from build123d import *

# Parameters (mm, degrees)
BOSS_EXTRU_1_DEPTH = 1.9


with BuildPart() as part:
    # Esquisse1 → Boss.-Extru.1 (new body)
    with BuildSketch(Plane.XY):
        with BuildLine():
            Line((103.141629659, -93.104422445), (-104.537862265, -93.104422445))
            add(Edge.make_bspline(
                [(-104.537862265, -93.104422445), (-104.576313156, -93.104422445), (-104.614764048, -93.104422445), (-104.653209533, -93.104125461), (-104.768513557, -93.101452602), (-104.883671631, -93.090761166), (-104.960260867, -93.08067219), (-105.150982063, -93.049552521), (-105.339086356, -93.007455152), (-105.450747192, -92.977883193), (-105.671146078, -92.909389067), (-105.884660771, -92.820748262), (-105.989422935, -92.771633631), (-106.194408631, -92.664300797), (-106.389220526, -92.539730583), (-106.48384332, -92.473274378), (-106.667043194, -92.332296267), (-106.837192824, -92.17573974), (-106.91879647, -92.093784348), (-107.074644208, -91.922954256), (-107.214938405, -91.739155447), (-107.281028071, -91.644254137), (-107.404754439, -91.448928258), (-107.51089869, -91.243516958), (-107.55945325, -91.138557181), (-107.64728317, -90.924663828), (-107.716066547, -90.703891793), (-107.745614057, -90.592075935), (-107.794855636, -90.366164197), (-107.824060167, -90.136851737), (-107.833655342, -90.021622167), (-107.842835855, -89.790570025), (-107.832005382, -89.559439241), (-107.821514669, -89.444212724), (-107.790403383, -89.216374252), (-107.738630165, -88.992714706), (-107.708207682, -88.882559264), (-107.650563592, -88.701220982), (-107.582401802, -88.523090493), (-107.553106564, -88.452964824), (-107.50557398, -88.350258026), (-107.451336724, -88.251263547), (-107.432968479, -88.218893501), (-107.414357288, -88.186657973), (-107.395746098, -88.154422445)],
                knots=[0, 0, 0, 0, 0, 0, 0.027851934, 0.027851934, 0.027851934, 0.083555801, 0.083555801, 0.083555801, 0.167111603, 0.167111603, 0.167111603, 0.250667404, 0.250667404, 0.250667404, 0.334223205, 0.334223205, 0.334223205, 0.417779006, 0.417779006, 0.417779006, 0.501334808, 0.501334808, 0.501334808, 0.584890609, 0.584890609, 0.584890609, 0.66844641, 0.66844641, 0.66844641, 0.752002212, 0.752002212, 0.752002212, 0.835558013, 0.835558013, 0.835558013, 0.918223942, 0.918223942, 0.918223942, 0.973037938, 0.973037938, 0.973037938, 1, 1, 1, 1, 1, 1], degree=5))
            Line((-107.395746098, -88.154422445), (-3.556000135, 91.701293407))
            add(Edge.make_bspline(
                [(-3.556000135, 91.701293407), (-3.53677469, 91.734592855), (-3.517549244, 91.767892304), (-3.498069305, 91.801038579), (-3.43810253, 91.899558363), (-3.371264438, 91.993942462), (-3.324232511, 92.055226199), (-3.201921489, 92.204835765), (-3.071411952, 92.346690177), (-2.989971465, 92.428605318), (-2.820454369, 92.585229289), (-2.636931834, 92.725818035), (-2.542016234, 92.791987415), (-2.346570425, 92.915843818), (-2.141283507, 93.022270761), (-2.036419348, 93.070988402), (-1.822728786, 93.159155091), (-1.602072042, 93.22823073), (-1.490294768, 93.257923864), (-1.264427699, 93.307476918), (-1.035106162, 93.337075852), (-0.919874384, 93.346860527), (-0.688854027, 93.356347766), (-0.457890497, 93.345565733), (-0.342715384, 93.335135327), (-0.113563347, 93.304251593), (0.112022532, 93.253433727), (0.223631661, 93.223114692), (0.443897755, 93.152803282), (0.657090436, 93.063438917), (0.761679759, 93.014133797), (0.96636704, 92.906558284), (1.161116934, 92.781613428), (1.255660668, 92.714914945), (1.437418929, 92.574052545), (1.605227169, 92.41738585), (1.685413339, 92.335961486), (1.813634853, 92.195371099), (1.933819487, 92.047276013), (1.979902479, 91.986842758), (2.045082883, 91.894324933), (2.103695988, 91.797856852), (2.122545148, 91.765764463), (2.141156339, 91.733528935), (2.159767529, 91.701293407)],
                knots=[0, 0, 0, 0, 0, 0, 0.027851934, 0.027851934, 0.027851934, 0.083555801, 0.083555801, 0.083555801, 0.167111603, 0.167111603, 0.167111603, 0.250667404, 0.250667404, 0.250667404, 0.334223205, 0.334223205, 0.334223205, 0.417779006, 0.417779006, 0.417779006, 0.501334808, 0.501334808, 0.501334808, 0.584890609, 0.584890609, 0.584890609, 0.66844641, 0.66844641, 0.66844641, 0.752002212, 0.752002212, 0.752002212, 0.835558013, 0.835558013, 0.835558013, 0.918223942, 0.918223942, 0.918223942, 0.973037938, 0.973037938, 0.973037938, 1, 1, 1, 1, 1, 1], degree=5))
            Line((2.159767529, 91.701293407), (105.997013492, -88.150092318))
            add(Edge.make_bspline(
                [(105.997013492, -88.150092318), (105.997513492, -88.150958343), (105.998013492, -88.151824369), (105.998513492, -88.152690394), (105.999013492, -88.15355642), (106.018738937, -88.187721894), (106.037964383, -88.221021342), (106.05692993, -88.254464601), (106.112267178, -88.355657245), (106.16058716, -88.46073278), (106.190144469, -88.532105492), (106.258554643, -88.712834727), (106.316149398, -88.896786508), (106.346369749, -89.008273609), (106.397251538, -89.233391706), (106.427243696, -89.462621256), (106.43709026, -89.577905267), (106.446630147, -89.809094504), (106.436155125, -90.040091661), (106.42591376, -90.155265507), (106.395423071, -90.384410308), (106.344915957, -90.610042473), (106.314742328, -90.721690999), (106.244722998, -90.942074145), (106.155695658, -91.155471889), (106.106553546, -91.260157873), (105.999259557, -91.464970991), (105.874440278, -91.659600259), (105.807819725, -91.75412963), (105.666497608, -91.937139248), (105.509695105, -92.107093417), (105.427633487, -92.188590241), (105.256608973, -92.344190568), (105.072620822, -92.484138664), (104.977626674, -92.550063114), (104.782119906, -92.673539742), (104.576539539, -92.77972567), (104.471505092, -92.828253704), (104.258635545, -92.915229776), (104.039054087, -92.982222627), (103.928445434, -93.010953705), (103.74257983, -93.0517016), (103.554233407, -93.081737003), (103.478855177, -93.091429417), (103.366142188, -93.101618391), (103.253291827, -93.104144789), (103.216074423, -93.104422445), (103.178852041, -93.104422445), (103.141629659, -93.104422445)],
                knots=[0, 0, 0, 0, 0, 0, 0.000723486, 0.000723486, 0.000723486, 0.000723486, 0.028555269, 0.028555269, 0.028555269, 0.084218835, 0.084218835, 0.084218835, 0.167714185, 0.167714185, 0.167714185, 0.251209535, 0.251209535, 0.251209535, 0.334704885, 0.334704885, 0.334704885, 0.418200235, 0.418200235, 0.418200235, 0.501695585, 0.501695585, 0.501695585, 0.585190935, 0.585190935, 0.585190935, 0.668686285, 0.668686285, 0.668686285, 0.752181634, 0.752181634, 0.752181634, 0.835676984, 0.835676984, 0.835676984, 0.918283106, 0.918283106, 0.918283106, 0.973057445, 0.973057445, 0.973057445, 1, 1, 1, 1, 1, 1], degree=5))
        make_face()
    extrude(amount=BOSS_EXTRU_1_DEPTH)


solid = part.part
Read the model definition and answer for the solid it produces. Units are mm, in the model's axes. Coordinates: 2 decimals unless noted, no trailing zeros. Loops run counter-clockwise (first coordinate to the right, second up) from the corner with the lowest first, then second, coordinate; pieces in that order, holes last. Notation, with made-up numbers: (32, 82.5) -> (80, 82.5) arc R23 ccw to (80, 99.5) -> close; hole circle Ø6 at (-6, -20). An arc over 180 degrees is marked (long way). Answer in a Markdown table with one row per item.
Item 1: A cutting plane is placed at A-A on y = -42. Determine the outline of the cut face in (x, z).
Returned:
| item | result |
|---|---|
| outline | (-80.75, 0) -> (79.35, 0) -> (79.35, 1.9) -> (-80.75, 1.9) -> close |
Item 2: A cutting plane is placed at B-B on x = -21. Determine the outline of the cut face in (y, z), plus the area to 3 significant figures.
Returned:
| item | result |
|---|---|
| outline | (-93.1, 0) -> (61.49, 0) -> (61.49, 1.9) -> (-93.1, 1.9) -> close |
| area | 294 mm^2 |
Item 3: Straight lines are drawn through the part: line 1 along X through (y, z) = (42, 0.95); line 2 along X through (y, z) = (58.5, 1.7); line 3 along Y through (x, z) = (71, 1.3). For each, find the intervals that lie inside material, in ascending order. Write a range as [from, to].
Returned:
| item | result |
|---|---|
| line 1 | x = [-32.25, 30.85] |
| line 2 | x = [-22.72, 21.33] |
| line 3 | y = [-93.1, -27.53] |
Item 4: This flat-tipped pin is pushed along its axis until it touches: P1, Ø1, axis at y = 30, z = 1, coming from the -X side. Where does it stop, or does it pass through?
Returned:
| item | result |
|---|---|
| P1 | stops at x = -39.47 |
